Input: part model. Units: mm. Frame: model coordinates. Face numbers are marked on the shaded views. Coordinates: 2 decimals unless noted, no trailing zeros. Loops run counter-clockwise (first coordinate to the right, second up) from the corner with the lowest first, then second, coordinate; pieces in that order, holes last. Notation, with made-up numbers: (11.25, 31) -> (19.25, 31) arc R20 cw to (19.25, 42) -> close; hole circle Ø4 at (88, 33). An arc over 180 degrees is marked (long way). Answer as a JSON object with one key per item and string values.
from build123d import *

# Parameters (mm, degrees)
F0_R     = 4.025
F1_DEPTH = 6.5
F0_R_2   = 7.5
F2_DEPTH = 3
F0_R_3   = 11
F3_DEPTH = 2
F4_R     = 0.99999


# Not quite as in the source:
# - a fillet or chamfer is up to 0.001 mm smaller than in the source, because OpenCascade refuses the exact size


with BuildPart() as f1:
    # F0 (on Top) → F1 (new body)
    with BuildSketch(Plane.XY):
        Circle(F0_R)
    extrude(amount=F1_DEPTH)

    # F0 (on Top) → F2 (join)
    with BuildSketch(Plane.XY):
        Circle(F0_R_2)
        Circle(F0_R, mode=Mode.SUBTRACT)
    extrude(amount=F2_DEPTH)

    # F0 (on Top) → F3 (join)
    with BuildSketch(Plane.XY):
        Circle(F0_R_3)
        Circle(F0_R_2, mode=Mode.SUBTRACT)
    extrude(amount=F3_DEPTH)

    # F4 (radius 1 in the source; OpenCascade refuses exactly that, so slightly less here)
    f4_edges = [f1.edges().sort_by_distance(p)[0] for p in [
        (-11, 0, 2),
        (-11, 0, 0),
    ]]
    fillet(f4_edges, radius=F4_R)


solid = f1.part
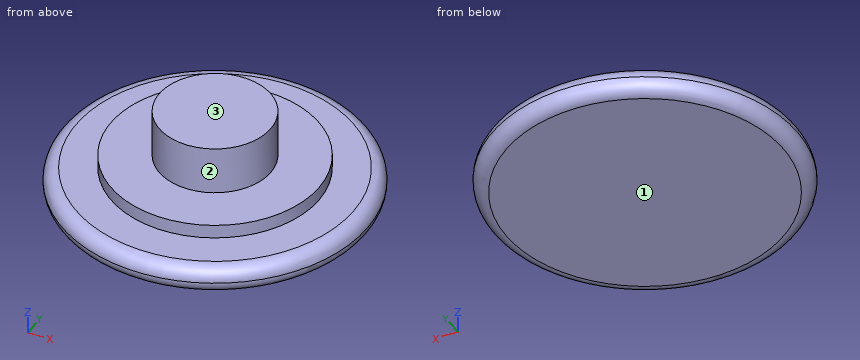
1. Line query: line 1 along Z through (x, y) = (7, 1.5); line 2 along Z through (x, y) = (7.75, -3); line 3 along X through (y, z) = (1.25, 4.5). Output: solid intervals per line, ascending.
Reply:
{"line 1": "z = 0 to 3", "line 2": "z = 0 to 2", "line 3": "x = -3.83 to 3.83"}
2. Pin query (flat end, axial travel): P1, Ø3, axis at x = -2.5, y = 7.5, coming from the +Z side; P2, Ø1.5, axis at y = 1.5, z = 5, coming from the +X side. Return the tip coordinate at first contact, or that it passes through.
Reply:
{"P1": "stops at z = 3", "P2": "stops at x = 3.95"}
3. Section query D-D (z = 0.5). Return loops of the section in (x, y).
Reply:
{"outline": "circle Ø21.73 at (0, 0)"}
4. Section query C-C (z = 5.5). Return loops of the section in (x, y) (3 decimals), plus the area to 3 significant figures.
Reply:
{"outline": "circle Ø8.05 at (0, 0)", "area": "50.9 mm2"}
5. Mould query, pull axis Z, two halves, no side actions, for the marked faces 1, 2 and 3. Classes: pulls with the +Z half, pulls with the -Z half, needs draft (parallel to the pull), parting line crosses it, or undercut.
Reply:
{"face 1": "pulls with the -Z half", "face 2": "needs draft", "face 3": "pulls with the +Z half"}
